```python
from build123d import *

# Parameters (mm, degrees)
SKETCH1_R           = 5.5
BOSS_EXTRUDE1_DEPTH = 0.76
SKETCH2_R           = 4.75
BOSS_EXTRUDE2_DEPTH = 3
SKETCH3_R           = 5.5
BOSS_EXTRUDE3_DEPTH = 0.76
SKETCH4_R           = 1.5
CUT_EXTRUDE1_DEPTH  = 4.52
SKETCH5_R           = 4.65
SKETCH5_R_2         = 2.35
CUT_EXTRUDE2_DEPTH  = 0.2
CUT_EXTRUDE3_START  = -0.2
SKETCH6_R           = 4.65
SKETCH6_R_2         = 2.35
CUT_EXTRUDE3_DEPTH  = 0.2


with BuildPart() as part:
    # Sketch1 → Boss-Extrude1 (new body)
    with BuildSketch(Plane(origin=(0, 0, 0), x_dir=(1, 0, 0), z_dir=(0, 1, 0))):
        with Locations(Location((0, 0, 0), (0, 0, 270))):
            Circle(SKETCH1_R)
    extrude(amount=BOSS_EXTRUDE1_DEPTH)

    # Sketch2 → Boss-Extrude2 (add)
    with BuildSketch(Plane(origin=(0, 0.76, 0), x_dir=(1, 0, 0), z_dir=(0, 1, 0))):
        with Locations(Location((0, 0, 0), (0, 0, 270))):
            Circle(SKETCH2_R)
    extrude(amount=BOSS_EXTRUDE2_DEPTH)

    # Sketch3 → Boss-Extrude3 (add)
    with BuildSketch(Plane(origin=(0, 3.76, 0), x_dir=(1, 0, 0), z_dir=(0, 1, 0))):
        with Locations(Location((0, 0, 0), (0, 0, 270))):
            Circle(SKETCH3_R)
    extrude(amount=BOSS_EXTRUDE3_DEPTH)

    # Sketch4 → Cut-Extrude1 (cut)
    with BuildSketch(Plane.XZ):
        with Locations(Location((0, 0, 0), (0, 0, 270))):
            Circle(SKETCH4_R)
    extrude(amount=-CUT_EXTRUDE1_DEPTH, mode=Mode.SUBTRACT)

    # Sketch5 → Cut-Extrude2 (cut)
    with BuildSketch(Plane(origin=(0, 4.52, 0), x_dir=(1, 0, 0), z_dir=(0, 1, 0))):
        with Locations(Location((0, 0, 0), (0, 0, 270))):
            Circle(SKETCH5_R)
        with Locations(Location((0, 0, 0), (0, 0, 270))):
            Circle(SKETCH5_R_2, mode=Mode.SUBTRACT)
    extrude(amount=-CUT_EXTRUDE2_DEPTH, mode=Mode.SUBTRACT)

    # Sketch6 → Cut-Extrude3 (cut)
    with BuildSketch(Plane.XZ.offset(CUT_EXTRUDE3_START)):
        with Locations(Location((0, 0, 0), (0, 0, 90))):
            Circle(SKETCH6_R)
        with Locations(Location((0, 0, 0), (0, 0, 90))):
            Circle(SKETCH6_R_2, mode=Mode.SUBTRACT)
    extrude(amount=CUT_EXTRUDE3_DEPTH, mode=Mode.SUBTRACT)


solid = part.part
```
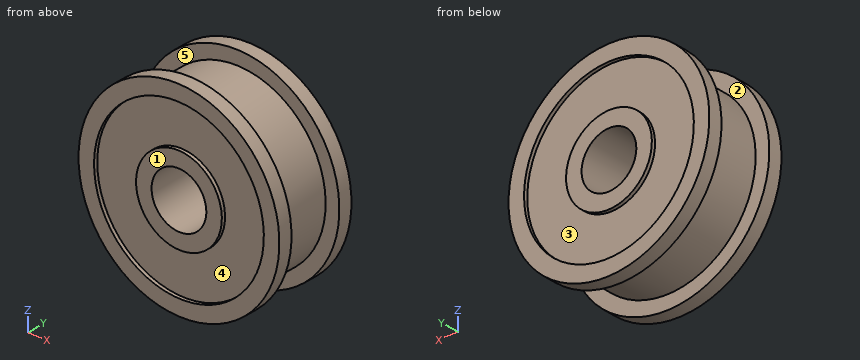
For this review, take the finished solid that the model builds, in its own axes (mm). Face numbers are marked on the shaded views. A direction names the side the tool comes from. Give positions to 0.01 mm unless a question says otherwise; leave off trailing zeros. Write each loop counter-clockwise with the first axis right and the second up, starting at its lowest first coordinate (ties: lowest second). Pieces come first, ordered by that corner, then holes. Notation, with made-up numbers: M 68,-20 L 105,-20 A13 ccw 105,-14 Z; hole C 68.25,5.5 d10. An arc over 180 degrees is marked long. One line per item, written item: value.
1) For P1, Ø1, axis at x = -0.5, y = 2, coming from the -Z side, flat-tipped, find the tip position at first contact; note if it passes through.
Results are:
P1: stops at z = -4.75
2) For line 1 (X direction, y = 0.1, z = 0); line 2 (X direction, y = 3.15, z = 0); line 3 (Y direction, x = -0.25, z = -5), list the stretches that pass through material, from the lowest coordinate up. Write a range as from..to.
Results are:
line 1: x = -5.5..-4.65, -2.35..-1.5, 1.5..2.35, 4.65..5.5
line 2: x = -4.75..-1.5, 1.5..4.75
line 3: y = 0..0.76, 3.76..4.52
3) The part is to be moulded in two halves that separate along Y. For the marked faces 3, 4 and 5, say which applies: +Y half, -Y half, draft (parallel to the pull), parting line (faces both ways), or undercut.
Results are:
face 3: +Y half
face 4: -Y half
face 5: undercut
4) For the marked faces 1 and 2, list the 3-axis set-ups (+Z, -Z, +X, -X, +Y, -Y) from which the entire face can be reached by the end or side of a thin tool; tool diameter is ignored.
Results are:
face 1: +Z, -Z, +X, -X, -Y
face 2: none
5) Take a section at D-D, the plane y = 3.15. Write out the cut boundary in (x, z), then the cut area to 3 significant figures.
Results are:
outline: C 0,0 d9.5; hole C 0,0 d3
area: 63.8 mm²
6) Take a section at C-C, the plane z = 2.75. Write out the cut boundary in (x, y), then the cut area to 3 significant figures.
Results are:
outline: M -4.76,0 L -3.75,0 L -3.75,0.2 L 3.75,0.2 L 3.75,0 L 4.76,0 L 4.76,0.76 L 3.87,0.76 L 3.87,3.76 L 4.76,3.76 L 4.76,4.52 L 3.75,4.52 L 3.75,4.32 L -3.75,4.32 L -3.75,4.52 L -4.76,4.52 L -4.76,3.76 L -3.87,3.76 L -3.87,0.76 L -4.76,0.76 Z
area: 34.7 mm²
